Input: part model. Units: mm. Frame: model coordinates. Face numbers are marked on the shaded views. A direction names the side the tool comes from. Round coordinates to 2 decimals unless told otherwise and drop trailing zeros. Order: outer loops, then holes, each group sorted by start corner. A loop starts at its lowest first (then second) coordinate and runs counter-clockwise, first axis right, second up. Notation, with made-up numbers: (53, 62.25) -> (58, 62.25) arc R9 ccw to (58, 78.25) -> close; hole circle Ø1 at (-18.5, -31). An arc over 180 degrees is marked (long way). Answer as CSV lines item,"result". Start each with the question number.
1) Section query C-C, the plane y = 24. Output: boundary loops of the cut face in (x, z), and give its area (3 significant figures).
2) Section query B-B, the plane z = 7.65. Output: boundary loops of the cut face in (x, y).
3) Section query A-A, the plane x = 68. Output: boundary loops of the cut face in (y, z).
4) Line query: L1, parallel to X at y = 19, z = 8; L2, parallel to Y at x = -47, z = 15; L3, parallel to X at y = 14.5, z = -7.5. Output: solid intervals per line, ascending.
5) First-contact query: P1, Ø5, axis at y = 27.5, z = 24, coming from the -X side; P2, Ø10, axis at x = -73.5, z = 14.5, coming from the -Y side; P3, Ø4, axis at x = -14, z = -21, coming from the +Y side; P4, Ø5, axis at y = 18.5, z = 2.5, coming from the -X side. Flat tips, straight axial feed; report the tip coordinate or a pass-through.
6) Mould query, pull axis X, two halves, no side actions, for the marked faces 3, 4 and 5. Classes: +X half, -X half, draft (parallel to the pull), parting line (faces both ways), or undercut.
7) Access query for the marked faces 1 and 2. Directions: +Z, -Z, +X, -X, +Y, -Y. A direction counts if a zero-diameter tool reaches every point of the face in a straight line with its end or side. Return the directions, or none.
8) Section query D-D, the plane x = 28.5. Output: boundary loops of the cut face in (y, z).
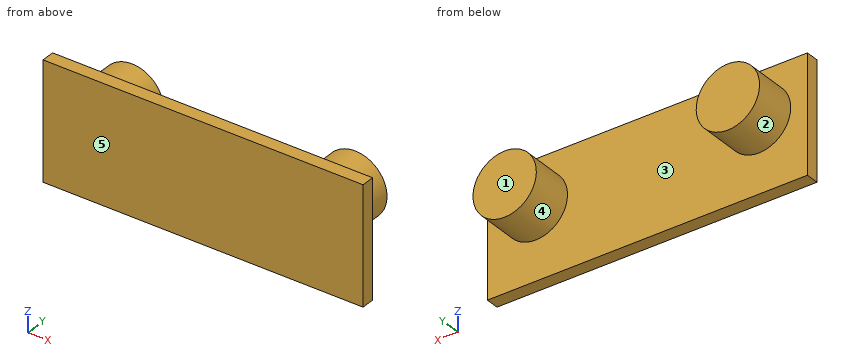
```python
from build123d import *

# Parameters (mm, degrees)
SKETCH_1_W      = 195
SKETCH_1_H      = 71.3
EXTRUDE_1_DEPTH = 8
SKETCH_2_R      = 19.3
EXTRUDE_2_DEPTH = 26


with BuildPart() as part:
    # 草图1 → 凸台-拉伸1 (new body)
    with BuildSketch(Plane(origin=(0, 0, 0), x_dir=(1, 0, 0), z_dir=(0, 1, 0))):
        Rectangle(SKETCH_1_W, SKETCH_1_H)
    extrude(amount=EXTRUDE_1_DEPTH)

    # 草图2 → 凸台-拉伸2 (add)
    with BuildSketch(Plane(origin=(0, 8, 0), x_dir=(1, 0, 0), z_dir=(0, 1, 0))):
        with Locations(Location((68, -7.65, 0), (0, 0, 90))):
            Circle(SKETCH_2_R)
        with Locations(Location((-68, -7.65, 0), (0, 0, 90))):
            Circle(SKETCH_2_R)
    extrude(amount=EXTRUDE_2_DEPTH)


solid = part.part
```
Findings:
1,outline,"circle Ø38.6 at (-68, 7.65); circle Ø38.6 at (68, 7.65)"
1,area,"2,340 mm^2"
2,outline,"(-97.5, 0) -> (97.5, 0) -> (97.5, 8) -> (87.3, 8) -> (87.3, 34) -> (48.7, 34) -> (48.7, 8) -> (-48.7, 8) -> (-48.7, 34) -> (-87.3, 34) -> (-87.3, 8) -> (-97.5, 8) -> close"
3,outline,"(0, -35.65) -> (8, -35.65) -> (8, -11.65) -> (34, -11.65) -> (34, 26.95) -> (8, 26.95) -> (8, 35.65) -> (0, 35.65) -> close"
4,L1,"x = -87.3 to -48.7, 48.7 to 87.3"
4,L2,"y = 0 to 8"
4,L3,"x = -79.96 to -56.04, 56.04 to 79.96"
5,P1,"stops at x = -81.44"
5,P2,"stops at y = 0"
5,P3,"stops at y = 8"
5,P4,"stops at x = -87.12"
6,face 3,"undercut"
6,face 4,"undercut"
6,face 5,"draft"
7,face 1,"+Z, -Z, +X, -X, +Y"
7,face 2,"+Y"
8,outline,"(0, -35.65) -> (8, -35.65) -> (8, 35.65) -> (0, 35.65) -> close"
